The model under review builds one solid part; all positions refer to its coordinate system, in mm. A direction names the side the tool comes from. Give positions to 0.01 mm unless a question says otherwise; leave off trailing zeros. Order: outer loops, then holes, each group sorted by start corner. A loop starts at its lowest first (then second) coordinate and runs counter-clockwise, first axis right, second up.
Autodesk Inventor part; units mm, degrees
ref_plane "YZ Plane" through (0, 0, 0) normal (1, 0, 0) x (0, 1, 0)
ref_plane "XZ Plane" through (0, 0, 0) normal (0, 1, 0) x (-1, 0, 0)
ref_plane "XY Plane" through (0, 0, 0) normal (0, 0, 1) x (1, 0, 0)
sketch "Sketch1" plane through (0, 0, 0) normal (0, 1, 0) x (-1, 0, 0)
  line L0 (300, -35) -> (300, -155)
  line L1 (220, -190) -> (220, -190)
  line L2 (255, -180) -> (255, -180)
  line L3 (245, -170) -> (240, -170)
  line L4 (230, -180) -> (230, -180)
  line L5 (220, -190) -> (220, -190)
  line L6 (185, -180) -> (185, -180)
  line L7 (195, -170) -> (200, -170)
  line L8 (210, -180) -> (210, -180)
  arc A0 (255, -172) -> (253, -170) centre (253, -172) ccw
  arc A1 (255, -180) -> (245, -170) centre (245, -180) ccw
  arc A2 (240, -170) -> (230, -180) centre (240, -180) ccw
  arc A3 (210, -180) -> (220, -190) centre (220, -180) ccw
  arc A4 (220, -190) -> (230, -180) centre (220, -180) ccw
  arc A5 (210, -180) -> (200, -170) centre (200, -180) ccw
  arc A6 (195, -170) -> (185, -180) centre (195, -180) ccw
  arc A7 (175, -190) -> (185, -180) centre (175, -180) ccw
  line L9 (265, -190) -> (265, -190)
  arc A8 (255, -180) -> (265, -190) centre (265, -180) ccw
  line L10 (220, 0) -> (220, 0)
  line L11 (255, -10) -> (255, -10)
  line L12 (245, -20) -> (240, -20)
  line L13 (230, -10) -> (230, -10)
  line L14 (220, 0) -> (220, 0)
  line L15 (185, -10) -> (185, -10)
  line L16 (195, -20) -> (200, -20)
  line L17 (210, -10) -> (210, -10)
  arc A9 (253, -20) -> (255, -18) centre (253, -18) ccw
  arc A10 (245, -20) -> (255, -10) centre (245, -10) ccw
  arc A11 (230, -10) -> (240, -20) centre (240, -10) ccw
  arc A12 (220, 0) -> (210, -10) centre (220, -10) ccw
  arc A13 (230, -10) -> (220, 0) centre (220, -10) ccw
  arc A14 (200, -20) -> (210, -10) centre (200, -10) ccw
  arc A15 (185, -10) -> (195, -20) centre (195, -10) ccw
  arc A16 (185, -10) -> (175, 0) centre (175, -10) ccw
  line L18 (265, 0) -> (265, 0)
  arc A17 (265, 0) -> (255, -10) centre (265, -10) ccw
  arc A18 (265, -190) -> (300, -155) centre (265, -155) ccw
  arc A19 (300, -35) -> (265, 0) centre (265, -35) ccw
  line L19 (175, 0) -> (365, 0) construction
  arc A20 (70, 0) -> (70, -190) centre (99.4643, -95) ccw
  line L20 (175, 0) -> (70, 0)
  line L21 (175, -190) -> (70, -190)
  point P0 (0, 0)
  point P1 (300, -190)
  point P2 (300, 0)
  point P3 (255, -170)
  point P4 (255, -190)
  point P5 (230, -170)
  point P6 (185, -170)
  point P7 (210, -170)
  point P8 (255, -20)
  point P9 (255, 0)
  point P10 (230, -20)
  point P11 (185, -20)
  point P12 (210, -20)
  point P13 (210, -10)
  dimension "d1" = 190
  dimension "d2" = 80
  dimension "d4" = 25
  dimension "d5" = 20
  dimension "d7" = 25
  dimension "d9" = 2
  dimension "d10" = 10
  dimension "d11" = 10
  dimension "d12" = 35
extrude "Extrusion1" add sketch "Sketch1" along normal blind 3
sketch "Sketch2" plane through (0, 3, 0) normal (0, 1, 0) x (1, 0, 0)
  arc A0 (-230, 10) -> (-210, 10) centre (-220, 10) ccw
  line L0 (-220, 0) -> (-220, 10)
  point P0 (0, 0)
sketch "Sketch3" plane through (0, 3, 0) normal (0, 1, 0) x (1, 0, 0)
  arc A0 (-245, 20) -> (-255, 10) centre (-245, 10) ccw
  arc A1 (-300, 35) -> (-265, 0) centre (-265, 35) ccw
  arc A2 (-245, 20) -> (-276.1181, 1.8128) centre (-249.7009, -7.6718) ccw
  line L0 (-276.1181, 1.8128) -> (-248.5566, -2.5367)
  line L1 (-248.5566, -2.5367) -> (-245, 20)
  arc A3 (-230, 10) -> (-210, 10) centre (-220, 10) ccw
  line L2 (-220, 0) -> (-220, 190)
  arc A4 (-210, 180) -> (-230, 180) centre (-220, 180) ccw
  arc A5 (-163.8819, 1.8128) -> (-195, 20) centre (-190.2991, -7.6718) ccw
  line L3 (-191.4434, -2.5367) -> (-195, 20)
  line L4 (-163.8819, 1.8128) -> (-191.4434, -2.5367)
  line L5 (-220, 95) -> (-300, 95)
  line L6 (-300, 155) -> (-300, 35)
  arc A6 (-276.1181, 188.1872) -> (-245, 170) centre (-249.7009, 197.6718) ccw
  line L7 (-276.1181, 188.1872) -> (-248.5566, 192.5367)
  line L8 (-248.5566, 192.5367) -> (-245, 170)
  arc A7 (-195, 170) -> (-163.8819, 188.1872) centre (-190.2991, 197.6718) ccw
  line L9 (-191.4434, 192.5367) -> (-195, 170)
  line L10 (-163.8819, 188.1872) -> (-191.4434, 192.5367)
  point P0 (0, 0)
extrude "Extrusion2" cut sketch "Sketch3" against normal blind 10
sketch "Sketch4" plane through (0, 3, 0) normal (0, 1, 0) x (1, 0, 0)
  line L0 (-300, 155) -> (-300, 35)
  line L1 (-300, 35) -> (-285, 35)
  line L2 (-285, 35) -> (-285, 25)
  circle A0 centre (-285, 25) radius 6.5
  line L3 (-300, 155) -> (-285, 155)
  line L4 (-300, 155) -> (-285, 155) construction
  line L5 (-285, 155) -> (-285, 165)
  circle A1 centre (-285, 165) radius 6.5
  point P0 (0, 0)
  dimension "d19" = 15
  dimension "d20" = 10
  dimension "d21" = 13
  dimension "d22" = 15
  dimension "d24" = 10
  dimension "d25" = 13
extrude "Extrusion3" cut sketch "Sketch4" against normal blind 10
sketch "Sketch5" plane through (0, 3, 0) normal (0, 1, 0) x (1, 0, 0)
  line L0 (-175.3338, 0.0056) -> (-163.8819, 1.8128)
  line L1 (-163.8819, 1.8128) -> (-179.2892, 1.8128)
  line L2 (-179.2892, 1.8128) -> (-179.2892, -4.2644)
  line L3 (-179.2892, -4.2644) -> (-163.8819, -4.2644)
  line L4 (-163.8819, -4.2644) -> (-163.8819, 1.8128)
  arc A0 (-300, 35) -> (-276.1181, 1.8128) centre (-265, 35) ccw
  line L5 (-276.1181, 1.8128) -> (-262.1006, 1.8128)
  line L6 (-262.1006, 1.8128) -> (-262.1006, -4.2644)
  line L7 (-262.1006, -4.2644) -> (-276.1181, -4.2644)
  line L8 (-276.1181, -4.2644) -> (-276.1181, 1.8128)
  line L9 (-163.8819, 188.1872) -> (-175.3338, 189.9944)
  line L10 (-163.8819, 188.1872) -> (-177.2047, 188.1872)
  line L11 (-177.2047, 188.1872) -> (-177.2047, 195.4302)
  line L12 (-177.2047, 195.4302) -> (-163.8819, 195.4302)
  line L13 (-163.8819, 195.4302) -> (-163.8819, 188.1872)
  arc A1 (-276.1181, 188.1872) -> (-245, 170) centre (-249.7009, 197.6718) ccw
  line L14 (-276.1181, 188.1872) -> (-262.1006, 188.1872)
  line L15 (-262.1006, 188.1872) -> (-262.1006, 191.8087)
  line L16 (-262.1006, 191.8087) -> (-276.1181, 191.8087)
  line L17 (-276.1181, 191.8087) -> (-276.1181, 188.1872)
  point P0 (0, 0)
extrude "Extrusion4" cut sketch "Sketch5" against normal blind 10
sketch "Sketch6" plane through (0, 3, 0) normal (0, 1, 0) x (1, 0, 0)
  arc A0 (-163.8819, 1.8128) -> (-195, 20) centre (-190.2991, -7.6718) ccw
  line L0 (-195, 20) -> (-173.6747, 14.9436)
  line L1 (-173.6747, 14.9436) -> (-195, 20)
  line L2 (-200, 20) -> (-195, 20)
  arc A1 (-173.6747, 14.9436) -> (-195, 20) centre (-187.6449, 3.5225) ccw
  arc A2 (-230, 10) -> (-210, 10) centre (-220, 10) ccw
  line L3 (-220, 0) -> (-220, 190)
  arc A3 (-210, 180) -> (-230, 180) centre (-220, 180) ccw
  line L4 (-300, 155) -> (-300, 35)
  line L5 (-300, 95) -> (0, 95)
  arc A4 (-245, 20) -> (-276.1181, 1.8128) centre (-249.7009, -7.6718) ccw
  line L6 (-245, 20) -> (-266.3253, 14.9436)
  line L7 (-266.3253, 14.9436) -> (-245, 20)
  arc A5 (-245, 20) -> (-266.3253, 14.9436) centre (-252.3551, 3.5225) ccw
  arc A6 (-195, 170) -> (-163.8819, 188.1872) centre (-190.2991, 197.6718) ccw
  line L8 (-195, 170) -> (-173.6747, 175.0564)
  line L9 (-173.6747, 175.0564) -> (-195, 170)
  line L10 (-200, 170) -> (-195, 170)
  arc A7 (-195, 170) -> (-173.6747, 175.0564) centre (-187.6449, 186.4775) ccw
  arc A8 (-210, 180) -> (-230, 180) centre (-220, 180) ccw
  line L11 (-220, 190) -> (-220, 0)
  arc A9 (-276.1181, 188.1872) -> (-245, 170) centre (-249.7009, 197.6718) ccw
  line L12 (-245, 170) -> (-266.3253, 175.0564)
  line L13 (-266.3253, 175.0564) -> (-245, 170)
  arc A10 (-266.3253, 175.0564) -> (-245, 170) centre (-252.3551, 186.4775) ccw
  point P0 (0, 0)
extrude "Extrusion5" cut sketch "Sketch6" against normal blind 10 contours L0 A0 | A0 A1 | A4 A5 | A6 A7 | A9 A10
sketch "Sketch7" plane through (0, 3, 0) normal (0, 1, 0) x (1, 0, 0)
  point P0 (0, 0)
properties part number "Onderplaat-v1"
Item 1: Clearance check with flat-ended pins moving along their axes: pin 1 Ø1.5 at (y, z) = (1.5, -22) entering from -X; pin 2 Ø0.9 at (y, z) = (1, -189) entering from -X; pin 3 Ø1.5 at (x, y) = (-266, 1.5) entering from -Z. State where each tip first meets the part, or that it passes through.
Values found:
pin 1: stops at x = -297.79
pin 2: stops at x = -225.19
pin 3: stops at z = -175.37
Item 2: For line 1 (Z direction, x = -285, y = 2.3); line 2 (Z direction, x = -188, y = 2.95); line 3 (X direction, y = 0.1, z = -26.5), list the stretches that pass through material, from the lowest coordinate up.
Values found:
line 1: z = -183.72 to -171.5, -158.5 to -31.5, -18.5 to -6.28
line 2: z = -168.44 to -21.56
line 3: x = -298.95 to -291.32, -278.68 to -27.35
Item 3: Take a section at A-A (x = -285). Give the boundary of the cut face in (y, z), and give its area (3 significant figures).
Values found:
outline: (0, -183.72) - (3, -183.72) - (3, -171.5) - (0, -171.5) - close; (0, -158.5) - (3, -158.5) - (3, -31.5) - (0, -31.5) - close; (0, -18.5) - (3, -18.5) - (3, -6.28) - (0, -6.28) - close
area: 454 mm2
Item 4: Take a section at B-B (z = -165). Give the boundary of the cut face in (x, y), and give its area (3 significant figures).
Values found:
outline: (-298.54, 0) - (-291.5, 0) - (-291.5, 3) - (-298.54, 3) - close; (-278.5, 0) - (-28.8, 0) - (-28.8, 3) - (-278.5, 3) - close
area: 770 mm2
Item 5: Take a section at D-D (z = -39). Give the boundary of the cut face in (x, y).
Values found:
outline: (-300, 0) - (-17.26, 0) - (-17.26, 3) - (-300, 3) - close
Item 6: Draft analysis for pull direction X (two halves, no side actions). For faces 4 (the cylindrical face through (-293.59, 1.48, -175.19)), 5 (the cylindrical face through (-183.32, 1.52, -21.04)), 6 (the flat face through (-148, 0, -94)), state which applies: released by +X, released by -X, zero draft, split by the parting line, or undercut.
Values found:
face 4: released by -X
face 5: undercut
face 6: zero draft
Item 7: Take a section at C-C (y = 1.7). Give the boundary of the cut face in (x, z), and give its area (3 significant figures).
Values found:
outline: (-300, -155) arc R35 ccw to (-276.12, -188.19) arc R28.07 cw to (-266.33, -175.06) arc R18.04 cw to (-245, -170) - (-240, -170) arc R10 cw to (-230, -180) arc R10 ccw to (-210, -180) arc R10 cw to (-200, -170) - (-195, -170) arc R18.04 cw to (-173.67, -175.06) arc R28.07 cw to (-163.88, -188.19) - (-163.88, -190) - (-70, -190) arc R99.46 ccw to (-70, 0) - (-163.88, 0) - (-163.88, -1.81) arc R28.07 cw to (-173.67, -14.94) arc R18.04 cw to (-195, -20) - (-200, -20) arc R10 cw to (-210, -10) arc R10 ccw to (-230, -10) arc R10 cw to (-240, -20) - (-245, -20) arc R18.04 cw to (-266.33, -14.94) arc R28.07 cw to (-276.12, -1.81) arc R35 ccw to (-300, -35) - close; hole circle Ø13 at (-285, -165); hole circle Ø13 at (-285, -25)
area: 49,400 mm2
Item 8: For faces 1 (the cylindrical face through (-278.8, 1.52, -26.95)), 2 (the cylindrical face through (-167.87, 1.52, -180.8)), 3 (the cylindrical face through (-272.13, 1.52, -9.2)), list the 3-axis set-ups (+Z, -Z, +X, -X, +Y, -Y) from which the entire face can be reached by the end or side of a thin tool; tool diameter is ignored.
Values found:
face 1: +Y, -Y
face 2: -Z, +Y, -Y
face 3: +Z, +Y, -Y
